For this review, take the finished solid that the model builds, in its own axes (mm). Face numbers are marked on the shaded views. Coordinates: 2 decimals unless noted, no trailing zeros. Loops run counter-clockwise (first coordinate to the right, second up) from the corner with the lowest first, then second, coordinate; pieces in that order, holes last.
1. Take a section at A-A, the plane y = 7.5. Count the separate pieces of the cut face and the enclosed holes in it, then the cut area to 3 significant figures.
2. To check wall thickness, follow probe 1 along Y at (x, z) = (-25, -1); probe 2 along Y at (x, z) = (20.5, 0). State the ranges of each line that lie inside material, in increasing order.
3. Take a section at B-B, the plane x = -7.5. State the section outline as (y, z) points (3 decimals), then the cut area to 3 significant figures.
4. Clearance check with flat-ended pins moving along their axes: P1, Ø0.6, axis at x = 11.5, z = -2, coming from the +Y side; P2, Ø2, axis at y = 6.5, z = 3.5, coming from the +X side. State where each tip first meets the part, or that it passes through.
5. Mouldability with a two-part tool opening along Y and no side actions: class the marked faces 1, 2, 3 and 4 as pulls with the +Y half, pulls with the -Y half, needs draft (parallel to the pull), parting line crosses it, or undercut.
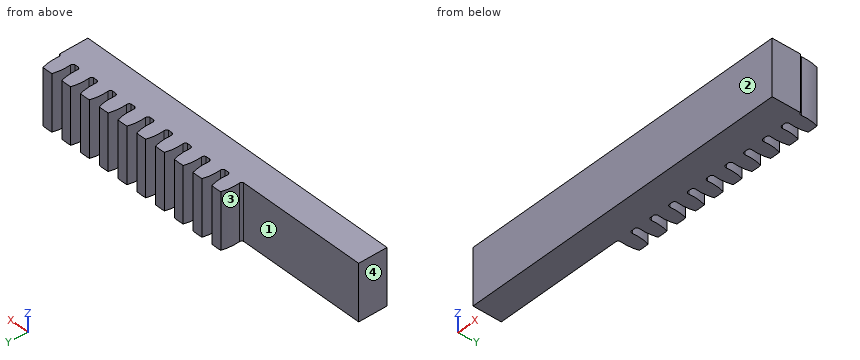
```python
from build123d import *

# Parameters (mm, degrees)
SKETCH1_W           = 59
SKETCH1_H           = 9.9
BOSS_EXTRUDE1_DEPTH = 5
BOSS_EXTRUDE4_DEPTH = 9.9


with BuildPart() as part:
    # Sketch1 → Boss-Extrude1 (new body)
    with BuildSketch(Plane(origin=(0, 0, 0), x_dir=(1, 0, 0), z_dir=(0, 1, 0))):
        with Locations((0, -0.405)):
            Rectangle(SKETCH1_W, SKETCH1_H)
    extrude(amount=BOSS_EXTRUDE1_DEPTH)

    # Sketch7 → Boss-Extrude4 (add, through all)
    with BuildSketch(Plane.XY.offset(5.355)):
        with BuildLine():
            Line((26.46999961, 4.995918044), (29.5, 4.995918044))
            ThreePointArc((29.5, 4.995918044), (29.231205307, 5.171705077), (29.148072876, 5.481931876))
            ThreePointArc((29.148072876, 5.481931876), (29.15553464, 7.003264285), (28.866052019, 8.496819705))
            ThreePointArc((28.866052019, 8.496819705), (27.984999805, 8.533849429), (27.103947591, 8.496819705))
            ThreePointArc((27.103947591, 8.496819705), (26.81446497, 7.003264285), (26.821926734, 5.481931876))
            ThreePointArc((26.821926734, 5.481931876), (26.738794303, 5.171705077), (26.46999961, 4.995918044))
        make_face()
        with BuildLine():
            Line((7.96999961, 4.995918044), (11, 4.995918044))
            ThreePointArc((11, 4.995918044), (10.731205307, 5.171705077), (10.648072876, 5.481931876))
            ThreePointArc((10.648072876, 5.481931876), (10.65553464, 7.003264285), (10.366052019, 8.496819705))
            ThreePointArc((10.366052019, 8.496819705), (9.484999805, 8.533849429), (8.603947591, 8.496819705))
            ThreePointArc((8.603947591, 8.496819705), (8.31446497, 7.003264285), (8.321926734, 5.481931876))
            ThreePointArc((8.321926734, 5.481931876), (8.238794303, 5.171705077), (7.96999961, 4.995918044))
        make_face()
        with BuildLine():
            Line((22.76999961, 4.995918044), (25.8, 4.995918044))
            ThreePointArc((25.8, 4.995918044), (25.531205307, 5.171705077), (25.448072876, 5.481931876))
            ThreePointArc((25.448072876, 5.481931876), (25.45553464, 7.003264285), (25.166052019, 8.496819705))
            ThreePointArc((25.166052019, 8.496819705), (24.284999805, 8.533849429), (23.403947591, 8.496819705))
            ThreePointArc((23.403947591, 8.496819705), (23.11446497, 7.003264285), (23.121926734, 5.481931876))
            ThreePointArc((23.121926734, 5.481931876), (23.038794303, 5.171705077), (22.76999961, 4.995918044))
        make_face()
        with BuildLine():
            Line((19.06999961, 4.995918044), (22.1, 4.995918044))
            ThreePointArc((22.1, 4.995918044), (21.831205307, 5.171705077), (21.748072876, 5.481931876))
            ThreePointArc((21.748072876, 5.481931876), (21.75553464, 7.003264285), (21.466052019, 8.496819705))
            ThreePointArc((21.466052019, 8.496819705), (20.584999805, 8.533849429), (19.703947591, 8.496819705))
            ThreePointArc((19.703947591, 8.496819705), (19.41446497, 7.003264285), (19.421926734, 5.481931876))
            ThreePointArc((19.421926734, 5.481931876), (19.338794303, 5.171705077), (19.06999961, 4.995918044))
        make_face()
        with BuildLine():
            Line((15.36999961, 4.995918044), (18.4, 4.995918044))
            ThreePointArc((18.4, 4.995918044), (18.131205307, 5.171705077), (18.048072876, 5.481931876))
            ThreePointArc((18.048072876, 5.481931876), (18.05553464, 7.003264285), (17.766052019, 8.496819705))
            ThreePointArc((17.766052019, 8.496819705), (16.884999805, 8.533849429), (16.003947591, 8.496819705))
            ThreePointArc((16.003947591, 8.496819705), (15.71446497, 7.003264285), (15.721926734, 5.481931876))
            ThreePointArc((15.721926734, 5.481931876), (15.638794303, 5.171705077), (15.36999961, 4.995918044))
        make_face()
        with BuildLine():
            Line((11.66999961, 4.995918044), (14.7, 4.995918044))
            ThreePointArc((14.7, 4.995918044), (14.431205307, 5.171705077), (14.348072876, 5.481931876))
            ThreePointArc((14.348072876, 5.481931876), (14.35553464, 7.003264285), (14.066052019, 8.496819705))
            ThreePointArc((14.066052019, 8.496819705), (13.184999805, 8.533849429), (12.303947591, 8.496819705))
            ThreePointArc((12.303947591, 8.496819705), (12.01446497, 7.003264285), (12.021926734, 5.481931876))
            ThreePointArc((12.021926734, 5.481931876), (11.938794303, 5.171705077), (11.66999961, 4.995918044))
        make_face()
        with BuildLine():
            Line((4.26999961, 4.995918044), (7.3, 4.995918044))
            ThreePointArc((7.3, 4.995918044), (7.031205307, 5.171705077), (6.948072876, 5.481931876))
            ThreePointArc((6.948072876, 5.481931876), (6.95553464, 7.003264285), (6.666052019, 8.496819705))
            ThreePointArc((6.666052019, 8.496819705), (5.784999805, 8.533849429), (4.903947591, 8.496819705))
            ThreePointArc((4.903947591, 8.496819705), (4.61446497, 7.003264285), (4.621926734, 5.481931876))
            ThreePointArc((4.621926734, 5.481931876), (4.538794303, 5.171705077), (4.26999961, 4.995918044))
        make_face()
        with BuildLine():
            Line((0.56999961, 4.995918044), (3.6, 4.995918044))
            ThreePointArc((3.6, 4.995918044), (3.331205307, 5.171705077), (3.248072876, 5.481931876))
            ThreePointArc((3.248072876, 5.481931876), (3.25553464, 7.003264285), (2.966052019, 8.496819705))
            ThreePointArc((2.966052019, 8.496819705), (2.084999805, 8.533849429), (1.203947591, 8.496819705))
            ThreePointArc((1.203947591, 8.496819705), (0.91446497, 7.003264285), (0.921926734, 5.481931876))
            ThreePointArc((0.921926734, 5.481931876), (0.838794303, 5.171705077), (0.56999961, 4.995918044))
        make_face()
        with BuildLine():
            Line((-3.13000039, 4.995918044), (-0.1, 4.995918044))
            ThreePointArc((-0.1, 4.995918044), (-0.368794693, 5.171705077), (-0.451927124, 5.481931876))
            ThreePointArc((-0.451927124, 5.481931876), (-0.44446536, 7.003264285), (-0.733947981, 8.496819705))
            ThreePointArc((-0.733947981, 8.496819705), (-1.615000195, 8.533849429), (-2.496052409, 8.496819705))
            ThreePointArc((-2.496052409, 8.496819705), (-2.78553503, 7.003264285), (-2.778073266, 5.481931876))
            ThreePointArc((-2.778073266, 5.481931876), (-2.861205697, 5.171705077), (-3.13000039, 4.995918044))
        make_face()
        with BuildLine():
            Line((-6.83000039, 4.995918044), (-3.8, 4.995918044))
            ThreePointArc((-3.8, 4.995918044), (-4.068794693, 5.171705077), (-4.151927124, 5.481931876))
            ThreePointArc((-4.151927124, 5.481931876), (-4.14446536, 7.003264285), (-4.433947981, 8.496819705))
            ThreePointArc((-4.433947981, 8.496819705), (-5.315000195, 8.533849429), (-6.196052409, 8.496819705))
            ThreePointArc((-6.196052409, 8.496819705), (-6.48553503, 7.003264285), (-6.478073266, 5.481931876))
            ThreePointArc((-6.478073266, 5.481931876), (-6.561205697, 5.171705077), (-6.83000039, 4.995918044))
        make_face()
    extrude(amount=-BOSS_EXTRUDE4_DEPTH)


solid = part.part
```
Results list:
1. separate pieces: 10
1. enclosed holes: 0
1. area: 219 mm2
2. probe 1: y = 0 to 5
2. probe 2: y = 0 to 8.53
3. outline: (0, -4.545) - (5, -4.545) - (5, 5.355) - (0, 5.355) - close
3. area: 49.5 mm2
4. P1: stops at y = 5.05
4. P2: stops at x = 29.19
5. face 1: pulls with the +Y half
5. face 2: pulls with the -Y half
5. face 3: undercut
5. face 4: needs draft
